Geometry check sheet. Reference: drawing and pictorial views, mm from the part's lowest x, y, z. A direction names the side the tool comes from. Coordinates: 2 decimals unless noted, no trailing zeros. Write each loop counter-clockwise with the first axis right and the second up, starting at its lowest first coordinate (ties: lowest second). Pieces come first, ordered by that corner, then holes.
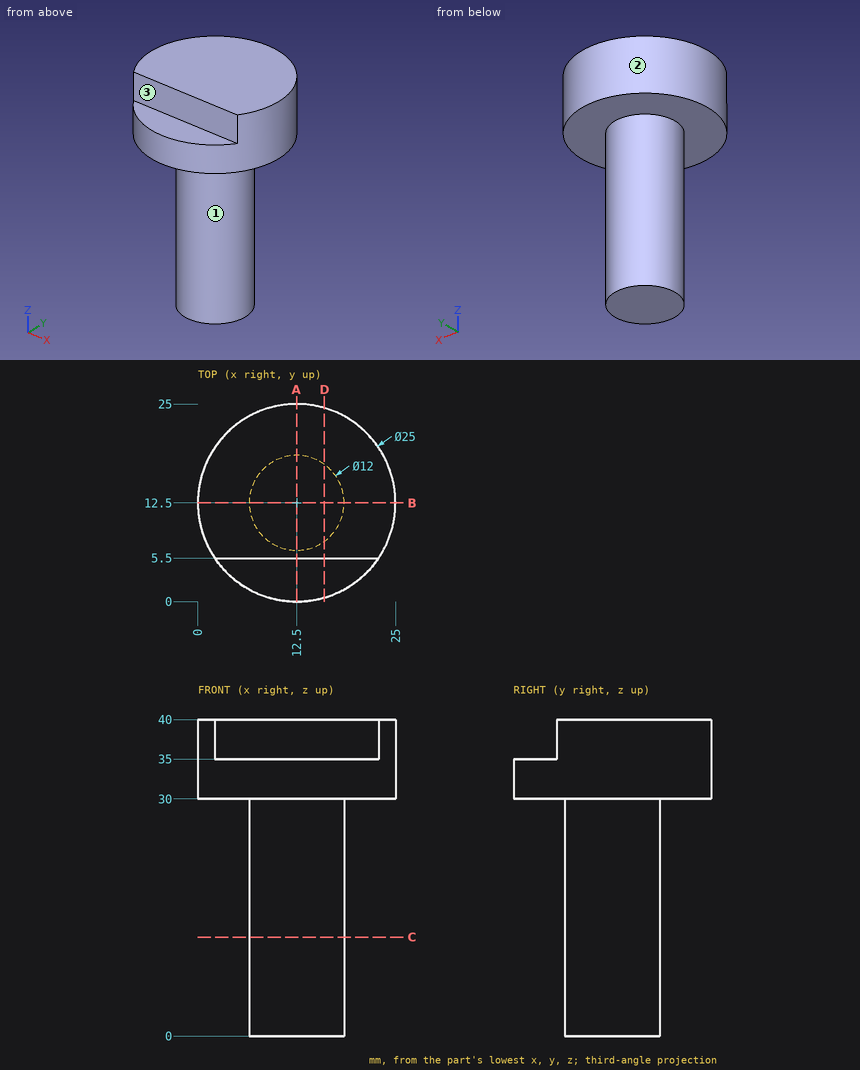
1. Sectioned sample at C-C, the plane z = 12.5. Record the boundary of the cut face in (x, y), and give its area (3 significant figures).
2. Sectioned sample at D-D, the plane x = 16. Record the boundary of the cut face in (y, z), and give its area (3 significant figures).
3. Material ranges on L1, parallel to Z at x = 5.75, y = 18.25; L2, parallel to Y at x = 17.5, z = 4; L3, parallel to Y at x = 8.5, z = 24.5, recorded low to high.
4. Sectioned sample at A-A, the plane x = 12.5. Record the boundary of the cut face in (y, z).
5. Gauge pin test, flat ends, axial feed: P1, Ø2, axis at y = 11, z = 6.5, coming from the +X side; P2, Ø4, axis at x = 10, y = 3, coming from the -Z side; P3, Ø6, axis at x = 7, z = 6, coming from the -Y side; P4, Ø4, axis at y = 22, z = 19, coming from the -X side. Record the tip position at first contact, or that the pin passes through.
6. Sectioned sample at B-B, the plane y = 12.5. Record the boundary of the cut face in (x, z).
7. Tool access check on the marked faces 1, 2 and 3. Record the directions out of +Z, -Z, +X, -X, +Y, -Y that give a thin tool (end or side, any length) a straight path to the whole face; none if there is none.
Outcome:
1. outline: circle Ø12 at (12.5, 12.5)
1. area: 113 mm2
2. outline: (0.5, 30) - (7.63, 30) - (7.63, 0) - (17.37, 0) - (17.37, 30) - (24.5, 30) - (24.5, 40) - (5.5, 40) - (5.5, 35) - (0.5, 35) - close
2. area: 507 mm2
3. L1: z = 30 to 40
3. L2: y = 9.18 to 15.82
3. L3: y = 8.03 to 16.97
4. outline: (0, 30) - (6.5, 30) - (6.5, 0) - (18.5, 0) - (18.5, 30) - (25, 30) - (25, 40) - (5.5, 40) - (5.5, 35) - (0, 35) - close
5. P1: stops at x = 18.48
5. P2: stops at z = 30
5. P3: stops at y = 7.05
5. P4: passes through
6. outline: (0, 30) - (6.5, 30) - (6.5, 0) - (18.5, 0) - (18.5, 30) - (25, 30) - (25, 40) - (0, 40) - close
7. face 1: -Z
7. face 2: +Z, -Z
7. face 3: +Z, +X, -X, -Y
